Design review of the part shown in the three views and the two pictorial views. Dimensions are in mm from the part's minimum x, y and z. A direction names the side the tool comes from. Coordinates: 2 decimals unless noted, no trailing zeros. Loops run counter-clockwise (first coordinate to the right, second up) from the corner with the lowest first, then second, coordinate; pieces in that order, holes last. Notation, with made-up numbers: (84.25, 48.5) - (88.25, 48.5) arc R10 cw to (88.25, 58.5) - close; hole circle Ø10 at (-8.5, -1). An arc over 180 degrees is marked (long way). One line per question, with ' | ' between items.
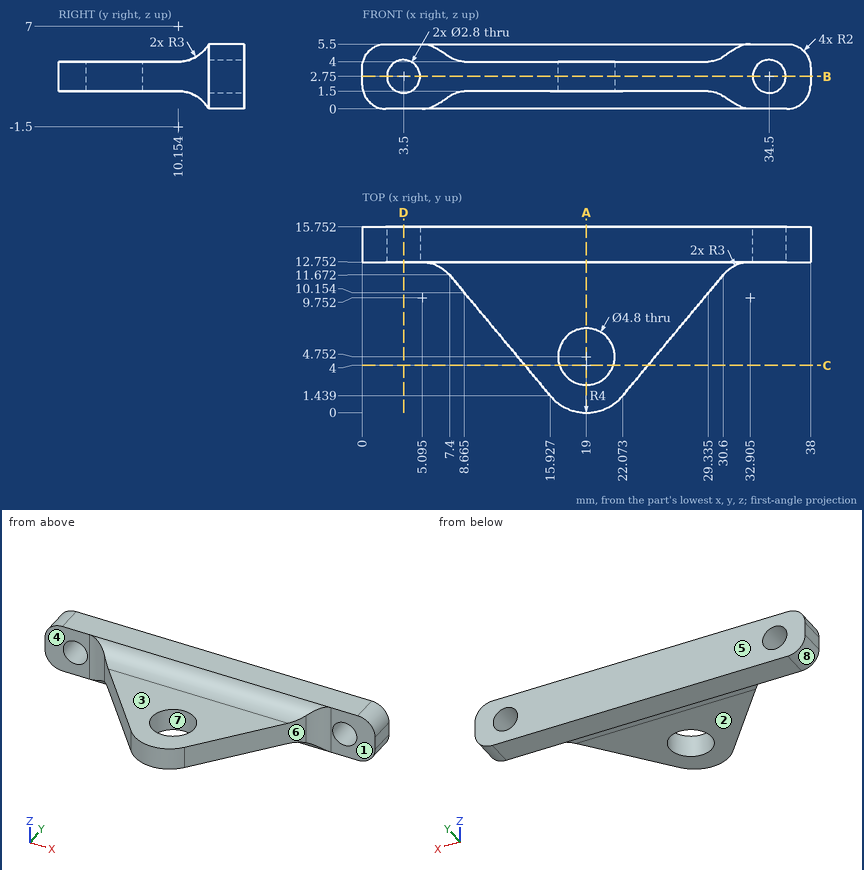
Q1. Take a section at B-B (z = 2.75). State how many separate pieces and enclosed holes the cut face has, plus the area to 3 significant figures.
Returned:
separate pieces: 3 | enclosed holes: 1 | area: 262 mm²
Q2. Take a section at D-D (x = 3.5). Give the boundary of the cut face in (y, z).
Returned:
outline: (12.75, 0) - (15.75, 0) - (15.75, 1.35) - (12.75, 1.35) - close; (12.75, 4.15) - (15.75, 4.15) - (15.75, 5.5) - (12.75, 5.5) - close
Q3. Tool access review of the marked faces 1, 2, 3 and 4: name each direction out of +Z, -Z, +X, -X, +Y, -Y from which nothing blocks a thin tool from reaching the whole face with its end or side.
Returned:
face 1: +Z, -Z, +X, -Y | face 2: -Z, +X, -X, -Y | face 3: +Z, +X, -X, -Y | face 4: +Z, -Z, -X, -Y
Q4. For pin 1 (1.5 mm diameter, centred on x = 35.5, z = 2, fed in from -Y); pin 2 (2 mm diameter, centred on y = 7.5, z = 1, fed in from -X) (1 decimal); pin 3 (1.5 mm diameter, centred on y = 7.5, z = 4.5, fed in from -X); pin 4 (1.7 mm diameter, centred on x = 34.5, z = 2.75, fed in from +Y), all flat-tipped, find the tip position at first contact; note any pin that passes through.
Returned:
pin 1: stops at y = 12.75 | pin 2: stops at x = 10.2 | pin 3: stops at x = 10.41 | pin 4: passes through
Q5. Draft analysis for pull direction X (two halves, no side actions). For the marked faces 5, 6, 7 and 8, state which applies: +X half, -X half, draft (parallel to the pull), parting line (faces both ways), or undercut.
Returned:
face 5: draft | face 6: +X half | face 7: undercut | face 8: -X half
Q6. Take a section at C-C (y = 4). Give the boundary of the cut face in (x, z).
Returned:
outline: (13.79, 1.5) - (16.72, 1.5) - (16.72, 4) - (13.79, 4) - close; (21.28, 1.5) - (24.21, 1.5) - (24.21, 4) - (21.28, 4) - close
Q7. Take a section at A-A (x = 19). Give the boundary of the cut face in (y, z).
Returned:
outline: (0, 1.5) - (2.35, 1.5) - (2.35, 4) - (0, 4) - close; (7.15, 1.5) - (10.15, 1.5) arc R3 cw to (12.75, 0) - (15.75, 0) - (15.75, 5.5) - (12.75, 5.5) arc R3 cw to (10.15, 4) - (7.15, 4) - close
Q8. To check wall thickness, follow line 1 along Z through (x, y) = (34.5, 15); line 2 along Z through (x, y) = (18, 2.25); line 3 along Y through (x, z) = (36.5, 3.9). State the ranges of each line that lie inside material, in increasing order.
Returned:
line 1: z = 0 to 1.35, 4.15 to 5.5 | line 2: z = 1.5 to 4 | line 3: y = 12.75 to 15.75
